Work out the finished part from the listing and answer in its coordinate system (mm). A direction names the side the tool comes from. Round coordinates to 2 decimals unless told otherwise and drop trailing zeros. Order: outer loops, then holes, each group sorted by start corner. A loop starts at its lowest first (then second) coordinate and runs counter-clockwise, first axis right, second up. Notation, with made-up numbers: (69, 73) -> (82, 73) arc R18 ccw to (82, 105) -> close; hole circle Ø11 at (-23.5, -5). An arc over 180 degrees is marked (long way). Use one line per item in the form item = value.
```python
from build123d import *

# Parameters (mm, degrees)
SKETCH1_R           = 15
BOSS_EXTRUDE1_DEPTH = 45
SKETCH2_R           = 10
CUT_EXTRUDE1_DEPTH  = 46
SKETCH3_R           = 14
BOSS_EXTRUDE2_DEPTH = 50
SKETCH5_R           = 10
CUT_EXTRUDE2_DEPTH  = 18


with BuildPart() as part:
    # Sketch1 → Boss-Extrude1 (new body)
    with BuildSketch(Plane.XY):
        Circle(SKETCH1_R)
    extrude(amount=BOSS_EXTRUDE1_DEPTH)

    # Sketch2 → Cut-Extrude1 (cut, through all)
    with BuildSketch(Plane(origin=(0, 0, 0), x_dir=(-1, 0, 0), z_dir=(0, 0, -1))):
        Circle(SKETCH2_R)
    extrude(amount=-CUT_EXTRUDE1_DEPTH, mode=Mode.SUBTRACT)

    # Sketch3 → Boss-Extrude2 (add)
    with BuildSketch(Plane(origin=(0, 0, 0), x_dir=(-1, 0, 0), z_dir=(0, 0, -1))):
        Circle(SKETCH3_R)
    extrude(amount=BOSS_EXTRUDE2_DEPTH)

    # Sketch5 → Cut-Extrude2 (cut)
    with BuildSketch(Plane(origin=(0, 0, -50), x_dir=(-1, 0, 0), z_dir=(0, 0, -1))):
        Circle(SKETCH5_R)
    extrude(amount=-CUT_EXTRUDE2_DEPTH, mode=Mode.SUBTRACT)


solid = part.part
```
Item 1: The part is cut by section C-C, the plane z = -42. Give the vertices of the cut face in (x, y).
Findings:
outline = circle Ø28 at (0, 0); hole circle Ø20 at (0, 0)
Item 2: The part is cut by section D-D, the plane z = -10. Give the vertices of the cut face in (x, y).
Findings:
outline = circle Ø28 at (0, 0)
Item 3: The part is cut by section A-A, the plane y = 0. Give the vertices of the cut face in (x, z), and give its area (3 significant figures).
Findings:
outline = (-15, 0) -> (-14, 0) -> (-14, -50) -> (-10, -50) -> (-10, -32) -> (10, -32) -> (10, -50) -> (14, -50) -> (14, 0) -> (15, 0) -> (15, 45) -> (10, 45) -> (10, 0) -> (-10, 0) -> (-10, 45) -> (-15, 45) -> close
area = 1,490 mm^2
Item 4: Determine the mould class of faces 4 (the flat face through (3, 10, -50)), 5 (the cylindrical face through (-14.985, 0.66, 22.185)), 6 (the flat face through (0, 0, -32)) for opening direction X: released by +X, released by -X, zero draft, split by the parting line, or undercut.
Findings:
face_4 = zero draft
face_5 = split by the parting line
face_6 = undercut
Item 5: Flat-ended cylindrical pins translate along their axes: P1, Ø6, axis at x = -6.5, z = 35.5, coming from the -Y side; P2, Ø2, axis at y = -7.5, z = 17, coming from the +X side; P3, Ø6, axis at x = -4.5, y = 4.5, coming from the -Z side. Find the tip coordinate at first contact, or state that the pin passes through.
Findings:
P1 = -14.59
P2 = 13.52
P3 = -32
Item 6: For faces 1 (the cylindrical face through (2.17, -9.76, -41.13)), 2 (the cylindrical face through (2.17, -9.76, 22.18)), 3 (the flat face through (3, -10, 45)), determine the directions among +Z, -Z, +X, -X, +Y, -Y from which every point of the face is accessible in a straight line to the end or side of a thin tool.
Findings:
face_1 = -Z
face_2 = +Z
face_3 = +Z, +X, -X, +Y, -Y
Item 7: Consider line 1 along Y through (x, z) = (0, -42.5); line 2 along Z through (x, y) = (-2.75, -7.5); line 3 along Z through (x, y) = (-7.25, -12.5). Determine where each line is inside the solid, lowest interval first.
Findings:
line_1 = -14 to -10, 10 to 14
line_2 = -32 to 0
line_3 = 0 to 45
